```python
from build123d import *

# Parameters (mm, degrees)
ESQUISSE1_R        = 3.9
BOSS_EXTRU_1_DEPTH = 9
CONG_1_R           = 3.9
BOSS_EXTRU_2_DEPTH = 2
ESQUISSE3_W        = 0.6
ESQUISSE3_H        = 0.6
BOSS_EXTRU_3_DEPTH = 4.9
ESQUISSE6_W        = 0.6
ESQUISSE6_H        = 0.6
BOSS_EXTRU_4_DEPTH = 5
ESQUISSE8_W        = 0.6
ESQUISSE8_H        = 0.6
BOSS_EXTRU_5_DEPTH = 5


with BuildPart() as part:
    # Esquisse1 → Boss.-Extru.1 (new body)
    with BuildSketch(Plane(origin=(0, 0, 0), x_dir=(1, 0, 0), z_dir=(0, 1, 0))):
        Circle(ESQUISSE1_R)
    extrude(amount=BOSS_EXTRU_1_DEPTH)

    # Congé1
    cong_1_edges = [part.edges().sort_by_distance(p)[0] for p in [
        (-3.9, 9, 0),
    ]]
    fillet(cong_1_edges, radius=CONG_1_R)

    # Esquisse2 → Boss.-Extru.2 (add)
    with BuildSketch(Plane.XZ):
        with BuildLine():
            Line((2.343608329, 3.9), (-2.343608329, 3.9))
            ThreePointArc((-2.343608329, 3.9), (0, -4.55), (2.343608329, 3.9))
        make_face()
    extrude(amount=BOSS_EXTRU_2_DEPTH)

    # Esquisse3 → Boss.-Extru.3 (add)
    with BuildSketch(Plane.XZ.offset(2)):
        with Locations((0, 0.275)):
            Rectangle(ESQUISSE3_W, ESQUISSE3_H)
        with Locations((0, -0.925)):
            Rectangle(ESQUISSE3_W, ESQUISSE3_H)
    extrude(amount=BOSS_EXTRU_3_DEPTH)

    # Esquisse6 → Boss.-Extru.4 (add)
    with BuildSketch(Plane(origin=(0, -2.123198642, 0.298396109), x_dir=(-1, 0, 0), z_dir=(0, -0.990268069, 0.139173101))):
        with Locations((0, -1.185218779)):
            Rectangle(ESQUISSE6_W, ESQUISSE6_H)
    extrude(amount=BOSS_EXTRU_4_DEPTH)

    # Esquisse8 → Boss.-Extru.5 (add)
    with BuildSketch(Plane(origin=(0, -2.212780783, -0.310986058), x_dir=(-1, 0, 0), z_dir=(0, -0.990268069, -0.139173101))):
        with Locations((0, 1.828893024)):
            Rectangle(ESQUISSE8_W, ESQUISSE8_H)
    extrude(amount=BOSS_EXTRU_5_DEPTH)


solid = part.part
```
Read the model definition and answer for the solid it produces. Units are mm, in the model's axes. A direction names the side the tool comes from. Give positions to 0.01 mm unless a question says otherwise; leave off trailing zeros. Order: outer loops, then holes, each group sorted by start corner. A loop starts at its lowest first (then second) coordinate and runs counter-clockwise, first axis right, second up.
(1) Given pin 1 (3 mm diameter, centred on x = 1.5, y = 5.5, fed in from -Z); pin 2 (0.6 mm diameter, centred on y = -3.5, z = 1.5, fed in from -X); pin 3 (1 mm diameter, centred on x = -2.5, z = -2.5, fed in from -Y), each flat-ended and moving along its own axis, determine where each tip first touches the part or whether it passes through.
(2) Find section D-D (y = 2.5). Give the vertices of the cut face in (x, z).
(3) Find section C-C (x = -3). Give the vertices of the cut face in (y, z), plus the area to 3 significant figures.
(4) For faces 1 (the flat face through (-0.3, -4.4, -2.5)), 2 (the flat face through (-1, 0, -4)), 3 (the flat face through (0.3, -4.4, 1.8)), determine the directions among +Z, -Z, +X, -X, +Y, -Y from which every point of the face is accessible in a straight line to the end or side of a thin tool.
(5) Find section A-A (y = -5). Give the vertices of the cut face in (x, z) (3 decimals), plus the area to 3 significant figures.
(6) Find section B-B (z = 1). Give the vertices of the cut face in (x, y).
(7) Straight lines are drawn through the part: L1, parallel to Y at x = -1.75, z = -3.75; L2, parallel to X at y = 6.5, z = 1.5; L3, parallel to Z at x = -3.25, y = 5. For each, find the intervals that lie inside material, in ascending order.
Result sheet:
1. pin 1: stops at z = -3.9
1. pin 2: stops at x = -0.3
1. pin 3: stops at y = -2
2. outline: circle Ø7.8 at (0, 0)
3. outline: (-2, -3.42) - (0, -3.42) - (0, -2.49) - (5.1, -2.49) arc R2.49 ccw to (5.1, 2.49) - (0, 2.49) - (0, 3.42) - (-2, 3.42) - close
3. area: 48.9 mm2
4. face 1: +Z, -Z, -X, -Y
4. face 2: +Y
4. face 3: +Z, -Z, +X, -Y
5. outline: (-0.3, -2.853) - (0.3, -2.853) - (0.3, -2.247) - (-0.3, -2.247) - close; (-0.3, -1.225) - (0.3, -1.225) - (0.3, -0.625) - (-0.3, -0.625) - close; (-0.3, -0.025) - (0.3, -0.025) - (0.3, 0.575) - (-0.3, 0.575) - close; (-0.3, 1.597) - (0.3, 1.597) - (0.3, 2.203) - (-0.3, 2.203) - close
5. area: 1.45 mm2
6. outline: (-4.44, -2) - (4.44, -2) - (4.44, 0) - (3.77, 0) - (3.77, 5.1) arc R3.77 ccw to (-3.77, 5.1) - (-3.77, 0) - (-4.44, 0) - close
7. L1: y = -2 to 0
7. L2: x = -3.32 to 3.32
7. L3: z = -2.16 to 2.16
